For this review, take the finished solid that the model builds, in its own axes (mm). A direction names the side the tool comes from. Coordinates: 2 decimals unless noted, no trailing zeros. Return JSON: item names as keys, results as strings.
```python
from build123d import *

# Parameters (mm, degrees)
F0_R     = 3
F0_R_2   = 2.5
F1_DEPTH = 740
F2_R     = 2
F3_R     = 7


# Not quite as in the source:
# - a feature names something its author has since deleted; it is built from what else it names


with BuildPart() as f1:
    # F0 (on Top) → F1 (new body)
    with BuildSketch(Plane.XY):
        with BuildLine():
            Line((18.15, -30), (30, -30))
            Line((30, -30), (30, -18.15))
            Line((30, -18.15), (27.5, -18.15))
            Line((27.5, -18.15), (27.5, -20.15))
            Line((27.5, -20.15), (21.5477069044, -20.15))
            ThreePointArc((21.5477069044, -20.15), (19.5, -15), (21.5477069044, -9.85))
            Line((21.5477069044, -9.85), (27.5, -9.85))
            Line((27.5, -9.85), (27.5, -11.85))
            Line((27.5, -11.85), (30, -11.85))
            Line((30, -11.85), (30, 11.85))
            Line((30, 11.85), (27.5, 11.85))
            Line((27.5, 11.85), (27.5, 9.85))
            Line((27.5, 9.85), (21.5477069044, 9.85))
            ThreePointArc((21.5477069044, 9.85), (19.5, 15), (21.5477069044, 20.15))
            Line((21.5477069044, 20.15), (27.5, 20.15))
            Line((27.5, 20.15), (27.5, 18.15))
            Line((27.5, 18.15), (30, 18.15))
            Line((30, 18.15), (30, 30))
            Line((30, 30), (18.15, 30))
            Line((18.15, 30), (18.15, 27.5))
            Line((18.15, 27.5), (20.15, 27.5))
            Line((20.15, 27.5), (20.15, 21.5477069044))
            ThreePointArc((20.15, 21.5477069044), (15, 19.5), (9.85, 21.5477069044))
            Line((9.85, 21.5477069044), (9.85, 27.5))
            Line((9.85, 27.5), (11.85, 27.5))
            Line((11.85, 27.5), (11.85, 30))
            Line((11.85, 30), (-11.85, 30))
            Line((-11.85, 30), (-11.85, 27.5))
            Line((-11.85, 27.5), (-9.85, 27.5))
            Line((-9.85, 27.5), (-9.85, 21.5477069044))
            ThreePointArc((-9.85, 21.5477069044), (-15, 19.5), (-20.15, 21.5477069044))
            Line((-20.15, 21.5477069044), (-20.15, 27.5))
            Line((-20.15, 27.5), (-18.15, 27.5))
            Line((-18.15, 27.5), (-18.15, 30))
            Line((-18.15, 30), (-30, 30))
            Line((-30, 30), (-30, 18.15))
            Line((-30, 18.15), (-27.5, 18.15))
            Line((-27.5, 18.15), (-27.5, 20.15))
            Line((-27.5, 20.15), (-21.5477069044, 20.15))
            ThreePointArc((-21.5477069044, 20.15), (-19.5, 15), (-21.5477069044, 9.85))
            Line((-21.5477069044, 9.85), (-27.5, 9.85))
            Line((-27.5, 9.85), (-27.5, 11.85))
            Line((-27.5, 11.85), (-30, 11.85))
            Line((-30, 11.85), (-30, -11.85))
            Line((-30, -11.85), (-27.5, -11.85))
            Line((-27.5, -11.85), (-27.5, -9.85))
            Line((-27.5, -9.85), (-21.5477069044, -9.85))
            ThreePointArc((-21.5477069044, -9.85), (-19.5, -15), (-21.5477069044, -20.15))
            Line((-21.5477069044, -20.15), (-27.5, -20.15))
            Line((-27.5, -20.15), (-27.5, -18.15))
            Line((-27.5, -18.15), (-30, -18.15))
            Line((-30, -18.15), (-30, -30))
            Line((-30, -30), (-18.15, -30))
            Line((-18.15, -30), (-18.15, -27.5))
            Line((-18.15, -27.5), (-20.15, -27.5))
            Line((-20.15, -27.5), (-20.15, -21.5477069044))
            ThreePointArc((-20.15, -21.5477069044), (-15, -19.5), (-9.85, -21.5477069044))
            Line((-9.85, -21.5477069044), (-9.85, -27.5))
            Line((-9.85, -27.5), (-11.85, -27.5))
            Line((-11.85, -27.5), (-11.85, -30))
            Line((-11.85, -30), (11.85, -30))
            Line((11.85, -30), (11.85, -27.5))
            Line((11.85, -27.5), (9.85, -27.5))
            Line((9.85, -27.5), (9.85, -21.5477069044))
            ThreePointArc((9.85, -21.5477069044), (15, -19.5), (20.15, -21.5477069044))
            Line((20.15, -21.5477069044), (20.15, -27.5))
            Line((20.15, -27.5), (18.15, -27.5))
            Line((18.15, -27.5), (18.15, -30))
        make_face()
        with Locations((-25, -25)):
            Circle(F0_R, mode=Mode.SUBTRACT)
        with Locations((-15, -15)):
            Circle(F0_R_2, mode=Mode.SUBTRACT)
        with Locations((25, -25)):
            Circle(F0_R, mode=Mode.SUBTRACT)
        with Locations((15, -15)):
            Circle(F0_R_2, mode=Mode.SUBTRACT)
        with Locations((-25, 25)):
            Circle(F0_R, mode=Mode.SUBTRACT)
        with Locations((-15, 15)):
            Circle(F0_R_2, mode=Mode.SUBTRACT)
        Polygon((-7, 22), (-7, 27.5), (0, 27.5), (7, 27.5), (7, 22), (10, 16), (10, 10), (16, 10), (22, 7), (27.5, 7), (27.5, 0), (27.5, -7), (22, -7), (16, -10), (10, -10), (10, -16), (7, -22), (7, -27.5), (0, -27.5), (-7, -27.5), (-7, -22), (-10, -16), (-10, -10), (-16, -10), (-22, -7), (-27.5, -7), (-27.5, 0), (-27.5, 7), (-22, 7), (-16, 10), (-10, 10), (-10, 16), align=None, mode=Mode.SUBTRACT)
        with Locations((15, 15)):
            Circle(F0_R_2, mode=Mode.SUBTRACT)
        with Locations((25, 25)):
            Circle(F0_R, mode=Mode.SUBTRACT)
    extrude(amount=F1_DEPTH)

    # F2
    f2_edges = [f1.edges().sort_by_distance(p)[0] for p in [
        (-7, 27.5, 370),
        (7, 27.5, 370),
    ]]
    fillet(f2_edges, radius=F2_R)

    # F3
    f3_edges = [f1.edges().sort_by_distance(p)[0] for p in [
        (-10, 16, 370),
        (10, 16, 370),
    ]]
    fillet(f3_edges, radius=F3_R)


solid = f1.part
```
1. We need section A-A (z = 142.5). Give the number of separate pieces and of enclosed holes in the cut face, plus the area to 3 significant figures.
Checks:
{"separate pieces": "1", "enclosed holes": "9", "area": "1,080 mm2"}
2. Wall thickness on L1, parallel to Y at x = 25, z = 393.5; L2, parallel to X at y = 24.5, z = 386; L3, parallel to X at y = -10.5, z = 463.5: over which ranges is each line inside the solid? List them lowest first. Write a range as from..to.
Checks:
{"L1": "-30..-28, -22..-20.15, -9.85..-7, 7..9.85, 20.15..22, 28..30", "L2": "-30..-27.96, -22.04..-20.15, -9.85..-7, 7..9.85, 20.15..22.04, 27.96..30", "L3": "-30..-27.5, -21..-10, 10..21, 27.5..30"}
3. For faces 1 (the face through (24, -30, 365)), 2 (the face through (0, -27.5, 365)), list the 3-axis set-ups (+Z, -Z, +X, -X, +Y, -Y) from which the entire face can be reached by the end or side of a thin tool; tool diameter is ignored.
Checks:
{"face 1": "+Z, -Z, +X, -X, -Y", "face 2": "+Z, -Z"}
4. Clearance check with a flat-ended pin moving along its axis: pin 1 Ø8 at (x, z) = (-14.5, 123.5) entering from -Y. State where the tip first meets the part, or that it passes through.
Checks:
{"pin 1": "y = -30"}
5. Draft analysis for pull direction X (two halves, no side actions). For faces 3 (the face through (27.5, 0, 365)), 4 (the face through (24, 30, 365)), 5 (the face through (-30, 0, 365)), state which applies: +X half, -X half, draft (parallel to the pull), parting line (faces both ways), or undercut.
Checks:
{"face 3": "undercut", "face 4": "draft", "face 5": "-X half"}
